```python
from build123d import *

# Parameters (mm, degrees)
SKETCH1_R           = 2.55
BOSS_EXTRUDE1_DEPTH = 2


with BuildPart() as part:
    # Sketch1 → Boss-Extrude1 (new body)
    with BuildSketch(Plane(origin=(0, 0, 0), x_dir=(1, 0, 0), z_dir=(0, 1, 0))):
        with BuildLine():
            Line((-288.144382289, 87.393439394), (-181.144388941, 87.393202129))
            ThreePointArc((-181.144388941, 87.393202129), (-179.023064297, 88.271879434), (-178.144382289, 90.393202129))
            Line((-178.144382289, 90.393202129), (-178.144382289, 120.393202129))
            Line((-178.144382289, 120.393202129), (271.855617711, 120.393202129))
            Line((271.855617711, 120.393202129), (271.855617711, -127.606797871))
            Line((271.855617711, -127.606797871), (-288.144382289, -127.606797871))
            Line((-288.144382289, -127.606797871), (-288.144382289, 87.393439394))
        make_face()
        with Locations((211.855617711, 110.393202129)):
            Circle(SKETCH1_R, mode=Mode.SUBTRACT)
        with Locations((-168.144382289, 110.393202129)):
            Circle(SKETCH1_R, mode=Mode.SUBTRACT)
        with Locations((21.855617711, 110.393202129)):
            Circle(SKETCH1_R, mode=Mode.SUBTRACT)
        with Locations((-238.144382289, -117.606797871)):
            Circle(SKETCH1_R, mode=Mode.SUBTRACT)
        with Locations((-84.811048956, -117.606797871)):
            Circle(SKETCH1_R, mode=Mode.SUBTRACT)
        with Locations((68.522284378, -117.606797871)):
            Circle(SKETCH1_R, mode=Mode.SUBTRACT)
        with Locations((221.855617711, -117.606797871)):
            Circle(SKETCH1_R, mode=Mode.SUBTRACT)
        with Locations((261.855617711, 0)):
            Circle(SKETCH1_R, mode=Mode.SUBTRACT)
        with Locations((-278.144382289, -2.55)):
            Circle(SKETCH1_R, mode=Mode.SUBTRACT)
    extrude(amount=BOSS_EXTRUDE1_DEPTH)


solid = part.part
```
Could you check a few things on this model? Use its own coordinates, in mm. Coordinates: 2 decimals unless noted, no trailing zeros. Write each loop counter-clockwise with the first axis right and the second up, starting at its lowest first coordinate (ties: lowest second). Pieces come first, ordered by that corner, then holes. Notation, with made-up numbers: M -1.75,28.25 L 16.25,28.25 A9 cw 16.25,38.25 Z; hole C -39.75,-19.75 d5. An arc over 180 degrees is marked long. Answer as CSV lines item,"result". Start each with the question number.
1) I want a section at A-A, the plane y = 1.1. Give the number of separate pieces and of enclosed holes in the cut face, and give its area (3 significant figures).
2) For P1, Ø6.5, axis at x = -84.81, z = 117.61, coming from the +Y side; P2, Ø1, axis at x = -211, y = 1.5, coming from the -Z side, each with a flat end and sliding along its axis, tell me the tip position at first contact or that it passes through.
3) I want a section at B-B, the plane z = -97.5. Please give me the cut outline in (x, y), and give its area (3 significant figures).
4) Please list where these lines run through material, in increasing order: line 1 (Z direction, x = 220, y = 1.4); line 2 (Z direction, x = -230, y = 1.9). Write a range as from..to.
Data:
1,separate pieces,"1"
1,enclosed holes,"9"
1,area,"135,000 mm^2"
2,P1,"stops at y = 2"
2,P2,"stops at z = -87.39"
3,outline,"M -178.14,0 L 271.86,0 L 271.86,2 L -178.14,2 Z"
3,area,"900 mm^2"
4,line 1,"z = -120.39..115.86, 119.36..127.61"
4,line 2,"z = -87.39..127.61"
